Part model, mm, in its own coordinate system. A direction names the side the tool comes from. Coordinates: 2 decimals unless noted, no trailing zeros. Write each loop counter-clockwise with the first axis right and the second up, starting at its lowest first coordinate (ties: lowest second). Pieces come first, ordered by that corner, then holes. Notation, with made-up numbers: (89.25, -20.75) -> (128.25, -20.75) arc R24 cw to (128.25, 1.25) -> close; hole circle Ø10 at (47, 60.5). An arc over 180 degrees is marked (long way). Write item = value, one per line.
Autodesk Fusion 360 part; units mm, degrees
sketch "01 - PRIMARY SUPPORT MECHANISM ( RIGHT SIDE ) SKETCH" plane through (0, 0, 0) normal (0, 0, 1) x (1, 0, 0)
  line L0 (-30, 35) -> (30, 35)
  line L1 (30, 35) -> (30, -35)
  line L2 (30, -35) -> (-30, -35)
  line L3 (-30, -35) -> (-30, 35)
  line L4 (-30, -19) -> (30, -19) construction
  line L5 (0, -35) -> (0, -5.422) construction
  line L6 (7.6, -5.422) -> (7.6, 0.1231)
  arc A0 (7.6, 0.1231) -> (-7.6, 0.1231) centre (0, 11.9996) ccw
  line L7 (-7.6, -5.422) -> (7.6, -5.422)
  line L8 (-7.6, -5.422) -> (-7.6, 0.1231)
  line L9 (4, -5.422) -> (4, -35)
  line L10 (-4, -5.422) -> (-4, -35)
  line L11 (-17.5, 11.9996) -> (17.5, 11.9996) construction
  circle A1 centre (17.5, 11.9996) radius 2.14
  line L12 (21.125, 14.0925) -> (17.5, 16.1854)
  line L13 (17.5, 16.1854) -> (13.875, 14.0925)
  line L14 (13.875, 14.0925) -> (13.875, 9.9067)
  line L15 (13.875, 9.9067) -> (17.5, 7.8138)
  line L16 (17.5, 7.8138) -> (21.125, 9.9067)
  line L17 (21.125, 9.9067) -> (21.125, 14.0925)
  line L18 (17.5, 11.9996) -> (17.5, 14.1396) construction
  circle A2 centre (-17.5, 11.9996) radius 2.14
  line L19 (-13.875, 9.9067) -> (-13.875, 14.0925)
  line L20 (-13.875, 14.0925) -> (-17.5, 16.1854)
  line L21 (-17.5, 16.1854) -> (-21.125, 14.0925)
  line L22 (-21.125, 14.0925) -> (-21.125, 9.9067)
  line L23 (-21.125, 9.9067) -> (-17.5, 7.8138)
  line L24 (-17.5, 7.8138) -> (-13.875, 9.9067)
  line L25 (-17.5, 11.9996) -> (-17.5, 14.1396) construction
  point P0 (17.5, 11.9996)
  point P1 (-17.5, 11.9996)
  dimension "d1" = 60
  dimension "d2" = 70
  dimension "d3" = 30
  dimension "d4" = 35
  dimension "d5" = 16
  dimension "d12" = 29.578
  dimension "d14" = 15.2
  dimension "d15" = 5.5451
  dimension "d16" = 14.1
  dimension "d21" = 17.4216
  dimension "d24" = 8
  dimension "d25" = 4
  dimension "d55" = 35
  dimension "d56" = 4.28
  dimension "d57" = 3.625
  dimension "d58" = 4.28
  dimension "d59" = 3.625
extrude "Extrude2" add sketch "01 - PRIMARY SUPPORT MECHANISM ( RIGHT SIDE ) SKETCH" along normal blind 12 contours L0 L1 L2 L3 L6 A0 L7 L8 L9 L10 L12 L13 L15 L16 L17 L20 L21 L22 L23 L24 | A0 L20 L21 L22 L23 L24 | A0 L12 L13 L15 L16 L17 | A1 | A2
extrude "Extrude3" add sketch "01 - PRIMARY SUPPORT MECHANISM ( RIGHT SIDE ) SKETCH" along normal blind 9 contours L2 L7 L9 L10
sketch "02 - PRIMARY SUPPORT MECHANISM ( RIGHT SIDE ) SKETCH" plane through (0, 0, 12) normal (0, 0, 1) x (-1, 0, 0)
  line L0 (7.6, 5.422) -> (7.6, -0.1231)
  arc A0 (-7.6, -0.1231) -> (7.6, -0.1231) centre (0, -11.9996) ccw
  line L1 (-7.6, -0.1231) -> (-7.6, 5.422)
  line L2 (-7.6, 5.422) -> (-4, 5.422)
  line L3 (-4, 5.422) -> (-4, 35)
  line L4 (-4, 35) -> (-30, 35)
  line L5 (-30, 35) -> (-30, -35)
  line L6 (-30, -35) -> (30, -35)
  line L7 (30, -35) -> (30, 35)
  line L8 (30, 35) -> (4, 35)
  line L9 (4, 35) -> (4, 5.422)
  line L10 (4, 5.422) -> (7.6, 5.422)
  line L11 (30, 35) -> (14, 35)
  line L12 (14, 35) -> (14, 19)
  line L13 (14, 19) -> (30, 19)
  line L14 (30, 19) -> (30, 35)
  line L15 (-30, 35) -> (-14, 35)
  line L16 (-14, 35) -> (-14, 19)
  line L17 (-14, 19) -> (-30, 19)
  line L18 (-30, 19) -> (-30, 35)
  dimension "d30" = 16
  dimension "d31" = 16
  dimension "d32" = 16
  dimension "d33" = 16
extrude "Extrude4" add sketch "02 - PRIMARY SUPPORT MECHANISM ( RIGHT SIDE ) SKETCH" along normal blind 45 contours L7 L8 L11 L12 L13 L14 | L4 L5 L15 L16 L17 L18
sketch "03 - PRIMARY SUPPORT MECHANISM ( RIGHT SIDE ) SKETCH" plane through (0, 0, 57) normal (0, 0, 1) x (-1, 0, 0)
  line L0 (-30, 19) -> (-14, 19)
  line L1 (-14, 19) -> (-14, 35)
  line L2 (-14, 35) -> (-30, 35)
  line L3 (-30, 35) -> (-30, 19)
  line L4 (-14, 27) -> (-30, 27) construction
  line L5 (-22, 19) -> (-22, 35) construction
  line L6 (-25.625, 24.9071) -> (-22, 22.8142)
  line L7 (-22, 22.8142) -> (-18.375, 24.9071)
  line L8 (-18.375, 24.9071) -> (-18.375, 29.0929)
  line L9 (-18.375, 29.0929) -> (-22, 31.1858)
  line L10 (-22, 31.1858) -> (-25.625, 29.0929)
  line L11 (-25.625, 29.0929) -> (-25.625, 24.9071)
  line L12 (-22, 22.8142) -> (-30, 22.8142)
  line L13 (-22, 31.1858) -> (-30, 31.1858)
  line L14 (-30, 31.1858) -> (-30, 22.8142)
  circle A0 centre (-22, 27) radius 3.625
  line L15 (-22, 23.375) -> (-22, 22.8142)
  line L16 (-22, 31.1858) -> (-22, 30.625)
  line L17 (-22, 23.375) -> (-30, 23.375)
  line L18 (-22, 30.625) -> (-30, 30.625)
  circle A1 centre (-22, 27) radius 2.14
  point P0 (-22, 27)
  dimension "d36" = 3.625
  dimension "d42" = 4.28
extrude "Extrude5" cut sketch "03 - PRIMARY SUPPORT MECHANISM ( RIGHT SIDE ) SKETCH" against normal blind 25 from surface at -6 contours L3 L6 L10 L11 L14 L17 L18 | L6 A0 L17 | A0 | L10 A0 L18 | L6 L11 A0 | L10 L11 A0 | A1
extrude "Extrude7" cut sketch "03 - PRIMARY SUPPORT MECHANISM ( RIGHT SIDE ) SKETCH" against normal blind 6 contours A1
sketch "04 - PRIMARY SUPPORT MECHANISM ( RIGHT SIDE ) SKETCH" plane through (0, 0, 57) normal (0, 0, 1) x (-1, 0, 0)
  line L0 (30, 19) -> (30, 35)
  line L1 (30, 35) -> (14, 35)
  line L2 (14, 35) -> (14, 19)
  line L3 (14, 19) -> (30, 19)
  line L4 (30, 27) -> (14, 27) construction
  line L5 (22, 35) -> (22, 19) construction
  line L6 (18.375, 24.9071) -> (22, 22.8142)
  line L7 (22, 22.8142) -> (25.625, 24.9071)
  line L8 (25.625, 24.9071) -> (25.625, 29.0929)
  line L9 (25.625, 29.0929) -> (22, 31.1858)
  line L10 (22, 31.1858) -> (18.375, 29.0929)
  line L11 (18.375, 29.0929) -> (18.375, 24.9071)
  circle A0 centre (22, 27) radius 3.625
  circle A1 centre (22, 27) radius 2.14
  line L12 (22, 22.8142) -> (30, 22.8142)
  line L13 (22, 31.1858) -> (30, 31.1858)
  line L14 (30, 31.1858) -> (30, 22.8142)
  line L15 (22, 23.375) -> (30, 23.375)
  line L16 (22, 30.625) -> (30, 30.625)
  point P0 (22, 27)
  dimension "d45" = 3.625
  dimension "d46" = 4.28
extrude "Extrude9" cut sketch "04 - PRIMARY SUPPORT MECHANISM ( RIGHT SIDE ) SKETCH" against normal blind 25 from surface at -6 contours L0 L7 L8 L9 L14 L15 L16 | L7 A0 L15 | A0 | L9 A0 L16 | L7 L8 A0 | L8 L9 A0 | A1
extrude "Extrude10" cut sketch "04 - PRIMARY SUPPORT MECHANISM ( RIGHT SIDE ) SKETCH" against normal blind 6 contours A1
extrude "Extrude11" cut sketch "01 - PRIMARY SUPPORT MECHANISM ( RIGHT SIDE ) SKETCH" along normal blind 12 contours A1 | A2
extrude "Extrude12" cut sketch "01 - PRIMARY SUPPORT MECHANISM ( RIGHT SIDE ) SKETCH" along normal blind 4 contours A0 L20 L21 L22 L23 L24 | A0 L12 L13 L15 L16 L17
Q1. Saw through at A-A on y = -27. Give the cut face in (x, z) (3 decimals).
Model answer:
outline = (-30, 0) -> (30, 0) -> (30, 26) -> (18.375, 26) -> (18.375, 51) -> (19.86, 51) -> (19.86, 57) -> (14, 57) -> (14, 12) -> (4, 12) -> (4, 9) -> (-4, 9) -> (-4, 12) -> (-14, 12) -> (-14, 57) -> (-19.86, 57) -> (-19.86, 51) -> (-18.375, 51) -> (-18.375, 26) -> (-30, 26) -> close; (-30, 51) -> (-24.14, 51) -> (-24.14, 57) -> (-30, 57) -> close; (24.14, 51) -> (30, 51) -> (30, 57) -> (24.14, 57) -> close
Q2. Which spindle directions (+Z, -Z, +X, -X, +Y, -Y) get a long thin tool onto all of the face, cutting with end or side? Do faces 5 (the face through (7.6, -3, 6)), 6 (the face through (22, -19, 34)), 7 (the face through (14, -27, 34)), 8 (the face through (-19.338, 8.875, 1.972)). Say none if no direction does.
Model answer:
face_5 = +Z, -Z
face_6 = +Z, +X, -X, +Y
face_7 = +Z, +Y, -Y
face_8 = -Z
Q3. Saw through at D-D on y = -8. Give the cut face in (x, z), and give its area (3 significant figures).
Model answer:
outline = (-30, 0) -> (30, 0) -> (30, 12) -> (4, 12) -> (4, 9) -> (-4, 9) -> (-4, 12) -> (-30, 12) -> close
area = 696 mm²
Q4. Saw through at C-C on x = -9. Give the cut face in (y, z).
Model answer:
outline = (-35, 0) -> (1.15, 0) -> (1.15, 12) -> (-35, 12) -> close; (22.85, 0) -> (35, 0) -> (35, 12) -> (22.85, 12) -> close
Q5. Pin check, flat tips, straight feed: pin 1 (1 mm diameter, centred on x = 23.5, y = -8, fed in from +Z); pin 2 (6 mm diameter, centred on x = -1, y = 20.5, fed in from +Z); pin 3 (2 mm diameter, centred on x = -21.5, y = -27.5, fed in from -Z); pin 4 (2.5 mm diameter, centred on x = -22, y = -27, fed in from +Z). Stop position of each tip, or through.
Model answer:
pin_1 = 12
pin_2 = through
pin_3 = 0
pin_4 = 26
Q6. Mould opens along Y. For faces 1 (the face through (-15.523, 12.819, 7.944)), 2 (the face through (-25, -27, 51)), 3 (the face through (0, 35, 6)), 4 (the face through (-30, -13, 11)) say: released by +Y, released by -Y, zero draft, split by the parting line, or undercut.
Model answer:
face_1 = undercut
face_2 = undercut
face_3 = released by +Y
face_4 = zero draft
Q7. Probe line 1 (X direction, y = -27, z = 53); line 2 (X direction, y = -19.5, z = 21); line 3 (Y direction, x = 18, z = 34.5). List the from-to ranges inside material, lowest first. Write a range as from..to.
Model answer:
line_1 = -30..-24.14, -19.86..-14, 14..19.86, 24.14..30
line_2 = -30..-14, 14..30
line_3 = -35..-19
Q8. Saw through at B-B on z = 25. Give the cut face in (x, y), and give its area (3 significant figures).
Model answer:
outline = (-30, -35) -> (-14, -35) -> (-14, -19) -> (-30, -19) -> close; (14, -35) -> (30, -35) -> (30, -19) -> (14, -19) -> close
area = 512 mm²
